Input: part model. Units: mm. Frame: model coordinates. Give positions to 0.01 mm unless a question says otherwise; leave off trailing zeros. Loops run counter-clockwise (first coordinate to the right, second up) from the corner with the lowest first, then second, coordinate; pieces in that order, holes last. Notation, with made-up numbers: (-9, -8) - (39, -8) arc R36 cw to (39, 26) - close; hole circle Ø3 at (-29, -31.75). An arc over 180 degrees is marked (long way). Answer as a JSON object with one key per item and string values.
from build123d import *

# Parameters (mm, degrees)
SKIZZE1_W                       = 250.4
SKIZZE1_H                       = 126.4
SKIZZE1_W_2                     = 248
SKIZZE1_H_2                     = 124
AUFSATZ_LINEAR_AUSTRAGEN1_DEPTH = 2.4
VERRUNDUNG1_R                   = 1
VERRUNDUNG2_R                   = 0.5
AUFSATZ_LINEAR_START            = -0.4
AUFSATZ_LINEAR_AUSTRAGEN2_DEPTH = 0.4
SKIZZE3_W                       = 246.4
SKIZZE3_H                       = 122.4
AUFSATZ_LINEAR_AUSTRAGEN3_DEPTH = 0.4
VERRUNDUNG3_R                   = 2


with BuildPart() as part:
    # Skizze1 → Aufsatz-Linear austragen1 (new body)
    with BuildSketch(Plane.XY):
        with Locations((125.2, -63.2)):
            Rectangle(SKIZZE1_W, SKIZZE1_H)
        with Locations((125.2, -63.2)):
            Rectangle(SKIZZE1_W_2, SKIZZE1_H_2, mode=Mode.SUBTRACT)
    extrude(amount=AUFSATZ_LINEAR_AUSTRAGEN1_DEPTH)

    # Verrundung1
    verrundung1_edges = [part.edges().sort_by_distance(p)[0] for p in [
        (1.2, -1.2, 1.2),
        (1.2, -125.2, 1.2),
        (249.2, -125.2, 1.2),
        (249.2, -1.2, 1.2),
        (0, 0, 1.2),
        (250.4, 0, 1.2),
        (250.4, -126.4, 1.2),
        (0, -126.4, 1.2),
    ]]
    fillet(verrundung1_edges, radius=VERRUNDUNG1_R)

    # Verrundung2
    verrundung2_edges = [part.edges().sort_by_distance(p)[0] for p in [
        (249.2, -63.2, 2.4),
        (125.2, -1.2, 2.4),
        (125.2, -125.2, 2.4),
        (250.4, -63.2, 2.4),
        (125.2, -126.4, 2.4),
        (0, -63.2, 2.4),
        (125.2, 0, 2.4),
        (1.2, -63.2, 2.4),
        (0.292893219, -0.292893219, 2.4),
        (0.292893219, -126.107106781, 2.4),
        (250.107106781, -0.292893219, 2.4),
        (250.107106781, -126.107106781, 2.4),
        (248.907106781, -1.492893219, 2.4),
        (248.907106781, -124.907106781, 2.4),
        (1.492893219, -124.907106781, 2.4),
        (1.492893219, -1.492893219, 2.4),
    ]]
    fillet(verrundung2_edges, radius=VERRUNDUNG2_R)

    # Skizze2 → Aufsatz-Linear austragen2 (add)
    with BuildSketch(Plane(origin=(0, 0, 0), x_dir=(-1, 0, 0), z_dir=(0, 0, -1)).offset(AUFSATZ_LINEAR_START)):
        with BuildLine():
            Line((-1, 1.2), (-249.4, 1.2))
            ThreePointArc((-249.4, 1.2), (-250.955634919, 0.555634919), (-251.6, -1))
            Line((-251.6, -1), (-251.6, -125.4))
            ThreePointArc((-251.6, -125.4), (-250.955634919, -126.955634919), (-249.4, -127.6))
            Line((-249.4, -127.6), (-1, -127.6))
            ThreePointArc((-1, -127.6), (0.555634919, -126.955634919), (1.2, -125.4))
            Line((1.2, -125.4), (1.2, -1))
            ThreePointArc((1.2, -1), (0.555634919, 0.555634919), (-1, 1.2))
        make_face()
        with BuildLine():
            Line((-250.4, -1), (-250.4, -125.4))
            ThreePointArc((-250.4, -125.4), (-250.107106781, -126.107106781), (-249.4, -126.4))
            Line((-249.4, -126.4), (-1, -126.4))
            ThreePointArc((-1, -126.4), (-0.292893219, -126.107106781), (0, -125.4))
            Line((0, -125.4), (0, -1))
            ThreePointArc((0, -1), (-0.292893219, -0.292893219), (-1, 0))
            Line((-1, 0), (-249.4, 0))
            ThreePointArc((-249.4, 0), (-250.107106781, -0.292893219), (-250.4, -1))
        make_face(mode=Mode.SUBTRACT)
    extrude(amount=AUFSATZ_LINEAR_AUSTRAGEN2_DEPTH)

    # Skizze3 → Aufsatz-Linear austragen3 (add)
    with BuildSketch(Plane(origin=(0, 0, 0), x_dir=(-1, 0, 0), z_dir=(0, 0, -1)).offset(AUFSATZ_LINEAR_START)):
        with BuildLine():
            Line((-1, 1.2), (-249.4, 1.2))
            ThreePointArc((-249.4, 1.2), (-250.955634919, 0.555634919), (-251.6, -1))
            Line((-251.6, -1), (-251.6, -125.4))
            ThreePointArc((-251.6, -125.4), (-250.955634919, -126.955634919), (-249.4, -127.6))
            Line((-249.4, -127.6), (-1, -127.6))
            ThreePointArc((-1, -127.6), (0.555634919, -126.955634919), (1.2, -125.4))
            Line((1.2, -125.4), (1.2, -1))
            ThreePointArc((1.2, -1), (0.555634919, 0.555634919), (-1, 1.2))
        make_face()
        with Locations((-125.2, -63.2)):
            Rectangle(SKIZZE3_W, SKIZZE3_H, mode=Mode.SUBTRACT)
    extrude(amount=AUFSATZ_LINEAR_AUSTRAGEN3_DEPTH)

    # Verrundung3
    verrundung3_edges = [part.edges().sort_by_distance(p)[0] for p in [
        (2, -124.4, 0.2),
        (248.4, -124.4, 0.2),
        (248.4, -2, 0.2),
        (2, -2, 0.2),
    ]]
    fillet(verrundung3_edges, radius=VERRUNDUNG3_R)


solid = part.part
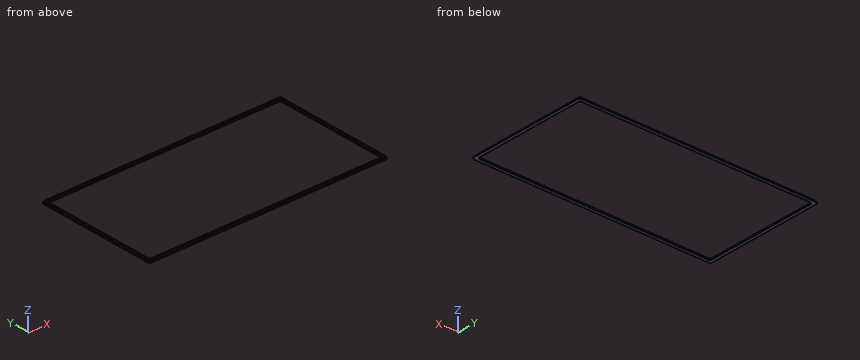
Item 1: Cut plane C-C (x = 161.5). Return loops of the section in (y, z).
Geometry check:
{"outline": "(-127.6, 0) - (-124.4, 0) - (-124.4, 0.4) - (-125.2, 0.4) - (-125.2, 1.9) arc R0.5 ccw to (-125.7, 2.4) - (-125.9, 2.4) arc R0.5 ccw to (-126.4, 1.9) - (-126.4, 0.4) - (-127.6, 0.4) - close; (-2, 0) - (1.2, 0) - (1.2, 0.4) - (0, 0.4) - (0, 1.9) arc R0.5 ccw to (-0.5, 2.4) - (-0.7, 2.4) arc R0.5 ccw to (-1.2, 1.9) - (-1.2, 0.4) - (-2, 0.4) - close"}
Item 2: Material intervals for line 1 (X direction, y = -107, z = 1); line 2 (Y direction, x = 165.5, z = 2.1); line 3 (X direction, y = -102, z = 0.15), sorted ascending. Write a range as [from, to].
Geometry check:
{"line 1": "x = [0, 1.2], [249.2, 250.4]", "line 2": "y = [-126.36, -125.24], [-1.16, -0.04]", "line 3": "x = [-1.2, 2], [248.4, 251.6]"}
Item 3: Contact query for flat-ended pins moving along their axis: P1, Ø0.8, axis at x = 136.5, z = 1, coming from the -Y side; P2, Ø0.8, axis at y = -68.5, z = 1.5, coming from the +X side. Output: stop coordinate, or through.
Geometry check:
{"P1": "stops at y = -126.4", "P2": "stops at x = 250.4"}
Item 4: Cut plane B-B (z = 1.15). Return loops of the section in (x, y).
Geometry check:
{"outline": "(0, -125.4) arc R1 ccw to (1, -126.4) - (249.4, -126.4) arc R1 ccw to (250.4, -125.4) - (250.4, -1) arc R1 ccw to (249.4, 0) - (1, 0) arc R1 ccw to (0, -1) - close; hole (1.2, -124.2) arc R1 ccw to (2.2, -125.2) - (248.2, -125.2) arc R1 ccw to (249.2, -124.2) - (249.2, -2.2) arc R1 ccw to (248.2, -1.2) - (2.2, -1.2) arc R1 ccw to (1.2, -2.2) - close"}
Item 5: Cut plane A-A (y = -42.5). Return loops of the section in (x, z).
Geometry check:
{"outline": "(-1.2, 0) - (2, 0) - (2, 0.4) - (1.2, 0.4) - (1.2, 1.9) arc R0.5 ccw to (0.7, 2.4) - (0.5, 2.4) arc R0.5 ccw to (0, 1.9) - (0, 0.4) - (-1.2, 0.4) - close; (248.4, 0) - (251.6, 0) - (251.6, 0.4) - (250.4, 0.4) - (250.4, 1.9) arc R0.5 ccw to (249.9, 2.4) - (249.7, 2.4) arc R0.5 ccw to (249.2, 1.9) - (249.2, 0.4) - (248.4, 0.4) - close"}
